Verification items for this drawing (mm, ordinates from the low corner). A direction names the side the tool comes from. Round coordinates to 2 decimals unless told otherwise and drop trailing zeros. Loops run counter-clockwise (first coordinate to the right, second up) from the corner with the lowest first, then second, coordinate; pieces in that order, holes last. Notation, with made-up numbers: (-5, -5) -> (53, -5) arc R22 ccw to (53, 26) -> close; hole circle Ø8 at (-26.75, 32.5). An arc over 180 degrees is marked (long way). Use a Markdown table: item, result. Add a question column.
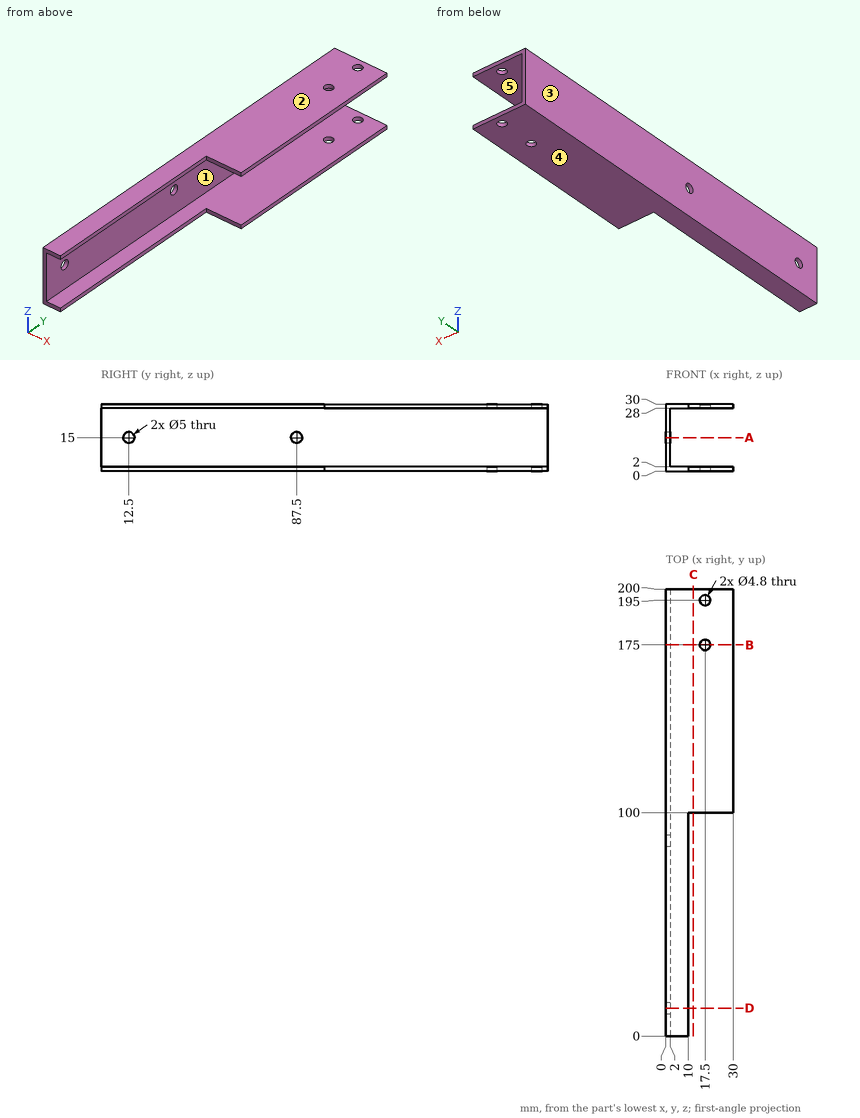
1) Sectioned sample at D-D on y = 12.5. Enter the section's corners in (x, z), then the cut area to 3 significant figures.
2) Access from +Z, -Z, +X, -X, +Y, -Y to the whole of each face (thin tool, end or side, straight path). Record for the marked faces 4 and 5.
3) Sectioned sample at C-C on x = 12.25. Enter the section's corners in (y, z), then the cut area to 3 significant figures.
4) Sectioned sample at A-A on z = 15. Enter the section's corners in (x, y).
5) Go/stop test with flat-tipped pins: pin 1 (1.6 mm diameter, centred on y = 55, z = 0.5, fed in from +X); pin 2 (6 mm diameter, centred on x = 17.5, y = 195, fed in from +Z); pin 3 (2 mm diameter, centred on x = 20, z = 1.5, fed in from -Y). Record where each tip stops, or that it passes through.
6) Sectioned sample at B-B on y = 175. Enter the section's corners in (x, z).
7) Thickness scan on line 1 (Y direction, x = 17.5, z = 1.45); line 2 (Z direction, x = 1, y = 87.5); line 3 (X direction, y = 195, z = 28.8). Record the ranges inside material, lowest first.
8) Release check for a two-part mould opening along Z. For the marked faces 1, 2 and 3 record: released by +Z, released by -Z, zero draft, split by the parting line, or undercut.
Geometry results:
| question | item | result |
|---|---|---|
| 1 | outline | (0, 0) -> (10, 0) -> (10, 2) -> (2, 2) -> (2, 12.5) -> (0, 12.5) -> close; (0, 17.5) -> (2, 17.5) -> (2, 28) -> (10, 28) -> (10, 30) -> (0, 30) -> close |
| 1 | area | 82.0 mm^2 |
| 2 | face 4 | -Z, +X, -X, +Y, -Y |
| 2 | face 5 | +X, +Y, -Y |
| 3 | outline | (100, 0) -> (200, 0) -> (200, 2) -> (100, 2) -> close; (100, 28) -> (200, 28) -> (200, 30) -> (100, 30) -> close |
| 3 | area | 400 mm^2 |
| 4 | outline | (0, 0) -> (2, 0) -> (2, 10) -> (0, 10) -> close; (0, 15) -> (2, 15) -> (2, 85) -> (0, 85) -> close; (0, 90) -> (2, 90) -> (2, 200) -> (0, 200) -> close |
| 5 | pin 1 | x = 10 |
| 5 | pin 2 | z = 30 |
| 5 | pin 3 | y = 100 |
| 6 | outline | (0, 0) -> (15.1, 0) -> (15.1, 2) -> (2, 2) -> (2, 28) -> (15.1, 28) -> (15.1, 30) -> (0, 30) -> close; (19.9, 0) -> (30, 0) -> (30, 2) -> (19.9, 2) -> close; (19.9, 28) -> (30, 28) -> (30, 30) -> (19.9, 30) -> close |
| 7 | line 1 | 100 to 172.6, 177.4 to 192.6, 197.4 to 200 |
| 7 | line 2 | 0 to 12.5, 17.5 to 30 |
| 7 | line 3 | 0 to 15.1, 19.9 to 30 |
| 8 | face 1 | undercut |
| 8 | face 2 | released by +Z |
| 8 | face 3 | zero draft |
